```python
from build123d import *

# Parameters (mm, degrees)
SKETCH1_R                       = 2.6
SKETCH1_R_2                     = 1.5
SKETCH1_W                       = 44.817241247
SKETCH1_H                       = 25.097655098
BOSS_EXTRUDE1_DEPTH             = 5
SKETCH2_R                       = 5
SKETCH2_R_2                     = 2.6
BOSS_EXTRUDE2_DEPTH             = 12
BOSS_EXTRUDE2_DIRECTION_2_REACH = 102.099
BOSS_EXTRUDE3_START             = -10
SKETCH3_R                       = 2.6
BOSS_EXTRUDE3_DEPTH             = 10


with BuildPart() as part:
    # Sketch1 → Boss-Extrude1 (new body)
    with BuildSketch(Plane.XY):
        with BuildLine():
            ThreePointArc((-87.127451531, -22.124820062), (-86.163911981, -24.765644938), (-83.600914186, -25.920377287))
            ThreePointArc((-83.600914186, -25.920377287), (-47.661538714, -29.763777863), (-13.512307499, -17.921462012))
            ThreePointArc((-13.512307499, -17.921462012), (-10.952947302, -16.861340184), (-9.892825615, -14.301979929))
            ThreePointArc((-9.892825615, -14.301979929), (8.007659225, 5.698020071), (-9.892825615, 25.698020071))
            ThreePointArc((-9.892825615, 25.698020071), (-10.952947373, 28.257380397), (-13.512307698, 29.317502154))
            ThreePointArc((-13.512307698, 29.317502154), (-47.63265011, 41.014505592), (-83.512307597, 37.317502154))
            ThreePointArc((-83.512307597, 37.317502154), (-86.071667988, 36.257380433), (-87.131789782, 33.698020071))
            ThreePointArc((-87.131789782, 33.698020071), (-90.927012387, 5.786304892), (-87.127451531, -22.124820062))
        make_face()
        with Locations((-83.512307698, -22.301979929)):
            Circle(SKETCH1_R, mode=Mode.SUBTRACT)
        with Locations((-83.512307698, 33.698020071)):
            Circle(SKETCH1_R, mode=Mode.SUBTRACT)
        with Locations((-13.512307698, 25.698020071)):
            Circle(SKETCH1_R, mode=Mode.SUBTRACT)
        with Locations((-13.512307698, -14.301979929)):
            Circle(SKETCH1_R, mode=Mode.SUBTRACT)
        with Locations((-85.16722268, 22.0113147)):
            Circle(SKETCH1_R_2, mode=Mode.SUBTRACT)
        with Locations((-85.523935714, -6.702744554)):
            Circle(SKETCH1_R_2, mode=Mode.SUBTRACT)
        with Locations((-6.064210345, 17.314888474)):
            Circle(SKETCH1_R_2, mode=Mode.SUBTRACT)
        with Locations((-5.445296778, -4.691116539)):
            Circle(SKETCH1_R_2, mode=Mode.SUBTRACT)
        with BuildLine():
            Line((-79.892825615, -14.301980328), (-79.892825615, -22.301979929))
            ThreePointArc((-79.892825615, -22.301979929), (-47.851158005, -23.48878534), (-17.131789782, -14.301980328))
            Line((-17.131789782, -14.301980328), (-79.892825615, -14.301980328))
        make_face(mode=Mode.SUBTRACT)
        with BuildLine():
            Line((-79.892825615, 33.698019868), (-79.892825615, 25.698020071))
            Line((-79.892825615, 25.698020071), (-17.131789782, 25.698020071))
            ThreePointArc((-17.131789782, 25.698020071), (-47.634119077, 36.587523584), (-79.892825615, 33.698019868))
        make_face(mode=Mode.SUBTRACT)
        with Locations((-48.117941597, 5.846082995)):
            Rectangle(SKETCH1_W, SKETCH1_H, mode=Mode.SUBTRACT)
    extrude(amount=BOSS_EXTRUDE1_DEPTH)

    # Sketch2 → Boss-Extrude2 (add)
    # profile 1 of 4: a face of its own
    with BuildSketch(Plane(origin=(0, 0, 0), x_dir=(-1, 0, 0), z_dir=(0, 0, -1))):
        with Locations((13.512307698, 25.698020071)):
            Circle(SKETCH2_R)
        with Locations((13.512307698, 25.698020071)):
            Circle(SKETCH2_R_2, mode=Mode.SUBTRACT)
    # profile 2 of 4: a face of its own
    with BuildSketch(Plane(origin=(0, 0, 0), x_dir=(-1, 0, 0), z_dir=(0, 0, -1))):
        with Locations((83.512307698, 33.698020071)):
            Circle(SKETCH2_R)
        with Locations((83.512307698, 33.698020071)):
            Circle(SKETCH2_R_2, mode=Mode.SUBTRACT)
    # profile 3 of 4: a face of its own
    with BuildSketch(Plane(origin=(0, 0, 0), x_dir=(-1, 0, 0), z_dir=(0, 0, -1))):
        with Locations((83.512307698, -22.301979929)):
            Circle(SKETCH2_R)
        with Locations((83.512307698, -22.301979929)):
            Circle(SKETCH2_R_2, mode=Mode.SUBTRACT)
    # profile 4 of 4: a face of its own
    with BuildSketch(Plane(origin=(0, 0, 0), x_dir=(-1, 0, 0), z_dir=(0, 0, -1))):
        with Locations((13.512307698, -14.301979929)):
            Circle(SKETCH2_R)
        with Locations((13.512307698, -14.301979929)):
            Circle(SKETCH2_R_2, mode=Mode.SUBTRACT)
    extrude(amount=BOSS_EXTRUDE2_DEPTH)

    # Boss-Extrude2 direction 2: up to this face of the body (flat: up to its plane)
    boss_extrude2_direction_2_end = Plane(part.part.faces().sort_by_distance((-86.07433416, -24.682416176, 5))[0])
    # Sketch2 → Boss-Extrude2 direction 2 (add, up to the picked face)
    with BuildSketch(Plane(origin=(0, 0, 0), x_dir=(-1, 0, 0), z_dir=(0, 0, -1)), mode=Mode.PRIVATE) as boss_extrude2_direction_2_sk1:
        with Locations((13.512307698, 25.698020071)):
            Circle(SKETCH2_R)
        with Locations((13.512307698, 25.698020071)):
            Circle(SKETCH2_R_2, mode=Mode.SUBTRACT)
    boss_extrude2_direction_2_tool1 = split(extrude(boss_extrude2_direction_2_sk1.sketch, amount=-BOSS_EXTRUDE2_DIRECTION_2_REACH, mode=Mode.PRIVATE), bisect_by=boss_extrude2_direction_2_end, keep=Keep.BOTH, mode=Mode.PRIVATE)
    # Sketch2 → Boss-Extrude2 direction 2 (add, up to the picked face)
    with BuildSketch(Plane(origin=(0, 0, 0), x_dir=(-1, 0, 0), z_dir=(0, 0, -1)), mode=Mode.PRIVATE) as boss_extrude2_direction_2_sk2:
        with Locations((83.512307698, 33.698020071)):
            Circle(SKETCH2_R)
        with Locations((83.512307698, 33.698020071)):
            Circle(SKETCH2_R_2, mode=Mode.SUBTRACT)
    boss_extrude2_direction_2_tool2 = split(extrude(boss_extrude2_direction_2_sk2.sketch, amount=-BOSS_EXTRUDE2_DIRECTION_2_REACH, mode=Mode.PRIVATE), bisect_by=boss_extrude2_direction_2_end, keep=Keep.BOTH, mode=Mode.PRIVATE)
    # Sketch2 → Boss-Extrude2 direction 2 (add, up to the picked face)
    with BuildSketch(Plane(origin=(0, 0, 0), x_dir=(-1, 0, 0), z_dir=(0, 0, -1)), mode=Mode.PRIVATE) as boss_extrude2_direction_2_sk3:
        with Locations((83.512307698, -22.301979929)):
            Circle(SKETCH2_R)
        with Locations((83.512307698, -22.301979929)):
            Circle(SKETCH2_R_2, mode=Mode.SUBTRACT)
    boss_extrude2_direction_2_tool3 = split(extrude(boss_extrude2_direction_2_sk3.sketch, amount=-BOSS_EXTRUDE2_DIRECTION_2_REACH, mode=Mode.PRIVATE), bisect_by=boss_extrude2_direction_2_end, keep=Keep.BOTH, mode=Mode.PRIVATE)
    # Sketch2 → Boss-Extrude2 direction 2 (add, up to the picked face)
    with BuildSketch(Plane(origin=(0, 0, 0), x_dir=(-1, 0, 0), z_dir=(0, 0, -1)), mode=Mode.PRIVATE) as boss_extrude2_direction_2_sk4:
        with Locations((13.512307698, -14.301979929)):
            Circle(SKETCH2_R)
        with Locations((13.512307698, -14.301979929)):
            Circle(SKETCH2_R_2, mode=Mode.SUBTRACT)
    boss_extrude2_direction_2_tool4 = split(extrude(boss_extrude2_direction_2_sk4.sketch, amount=-BOSS_EXTRUDE2_DIRECTION_2_REACH, mode=Mode.PRIVATE), bisect_by=boss_extrude2_direction_2_end, keep=Keep.BOTH, mode=Mode.PRIVATE)
    add(boss_extrude2_direction_2_tool1.solids().sort_by(Axis((-8.653729, 25.69802, 0), (0, 0, 1)))[0])
    add(boss_extrude2_direction_2_tool2.solids().sort_by(Axis((-78.653729, 33.69802, 0), (0, 0, 1)))[0])
    add(boss_extrude2_direction_2_tool3.solids().sort_by(Axis((-78.653729, -22.30198, 0), (0, 0, 1)))[0])
    add(boss_extrude2_direction_2_tool4.solids().sort_by(Axis((-8.653729, -14.30198, 0), (0, 0, 1)))[0])

    # Sketch3 → Boss-Extrude3 (add)
    with BuildSketch(Plane.XY.offset(5).offset(BOSS_EXTRUDE3_START)):
        with Locations(Location((-83.512307698, 33.698020071, 0), (0, 0, 180))):
            Circle(SKETCH3_R)
        with Locations(Location((-13.512307698, 25.698020071, 0), (0, 0, 180))):
            Circle(SKETCH3_R)
        with Locations(Location((-13.512307698, -14.301979929, 0), (0, 0, 180))):
            Circle(SKETCH3_R)
        with Locations(Location((-83.512307698, -22.301979929, 0), (0, 0, 180))):
            Circle(SKETCH3_R)
    extrude(amount=BOSS_EXTRUDE3_DEPTH)


solid = part.part
```
Geometry: final body of the model. Coordinates: model frame, mm. A direction names the side the tool comes from. Coordinates: 2 decimals unless noted, no trailing zeros. Order: outer loops, then holes, each group sorted by start corner. A loop starts at its lowest first (then second) coordinate and runs counter-clockwise, first axis right, second up. Notation, with made-up numbers: (2.25, -39.5) - (26.25, -39.5) arc R11 ccw to (26.25, -24.5) - close; hole circle Ø9 at (26, 54). An arc over 180 degrees is marked (long way). Return JSON: item names as keys, results as strings. Group by question number.
1. Cut plane A-A (x = -66.5). Output: boundary loops of the cut face in (y, z), plus the area to 3 significant figures.
2. Pull-direction query (X, two-part tool) for faces 1 (the face through (-83, -22, -5)), 2 (the face through (-86, 32, -12)), 3 (the face through (-13, 26, -5)), 4 (the face through (8.004, 5.306, 2.465)); classes: pulls with the +X half, pulls with the -X half, needs draft (parallel to the pull), parting line crosses it, or undercut.
3. Set-up query: faces 5 (the face through (-15.99, 26.48, -8.45)), 6 (the face through (-16, -16, -12)), 7 (the face through (-79.893, 28, 2)). Return all of +Z, -Z, +X, -X, +Y, -Y with unobstructed straight access to the full face (end or side cutting, diameter ignored); none if empty.
4. Cut plane D-D (x = -54.5). Output: boundary loops of the cut face in (y, z), plus the area to 3 significant figures.
5. Material intervals for line 1 along Y through (x, z) = (-49, 1); line 2 along Y through (x, z) = (-78, 1.5); line 3 along Y through (x, z) = (-84, -5.5), sorted ascending. Write a range as [from, to].
6. Cut plane B-B (z = -8). Output: boundary loops of the cut face in (x, y), plus the area to 3 significant figures.
7. Cut plane C-C (y = 14). Output: boundary loops of the cut face in (x, z).
8. Pin query (flat end, axial travel): pin 1 (4 mm diameter, centred on x = -51, z = 3, fed in from -Y); pin 2 (10 mm diameter, centred on x = -31, z = 0.5, fed in from -Y); pin 3 (1 mm diameter, centred on y = 24, z = -3.5, fed in from -X); pin 4 (8 mm diameter, centred on y = -2.5, z = -4.5, fed in from +X). Return the tip coordinate at first contact, or that it passes through.
Resolved:
{
 "1": {"outline": "(-29.76, 0) - (-24.08, 0) - (-24.08, 5) - (-29.76, 5) - close; (-14.3, 0) - (-6.7, 0) - (-6.7, 5) - (-14.3, 5) - close; (18.39, 0) - (25.7, 0) - (25.7, 5) - (18.39, 5) - close; (36.62, 0) - (41.04, 0) - (41.04, 5) - (36.62, 5) - close", "area": "125 mm²"},
 "2": {"face 1": "undercut", "face 2": "needs draft", "face 3": "undercut", "face 4": "pulls with the +X half"},
 "3": {"face 5": "-Z", "face 6": "-Z, +X, -X, +Y, -Y", "face 7": "+Z, -Z"},
 "4": {"outline": "(-30.26, 0) - (-24.11, 0) - (-24.11, 5) - (-30.26, 5) - close; (-14.3, 0) - (-6.7, 0) - (-6.7, 5) - (-14.3, 5) - close; (18.39, 0) - (25.7, 0) - (25.7, 5) - (18.39, 5) - close; (37.15, 0) - (41.52, 0) - (41.52, 5) - (37.15, 5) - close", "area": "127 mm²"},
 "5": {"line 1": "y = [-29.91, -23.63], [-14.3, -6.7], [18.39, 25.7], [36.75, 41.16]", "line 2": "y = [-27.6, -22.67], [-14.3, 25.7], [34.27, 38.93]", "line 3": "y = [-27.28, -24.86], [-19.75, -17.33], [28.72, 31.14], [36.25, 38.67]"},
 "6": {"outline": "circle Ø10 at (-83.51, -22.3); circle Ø10 at (-83.51, 33.7); circle Ø10 at (-13.51, -14.3); circle Ø10 at (-13.51, 25.7); hole circle Ø5.2 at (-83.51, -22.3); hole circle Ø5.2 at (-83.51, 33.7); hole circle Ø5.2 at (-13.51, -14.3); hole circle Ø5.2 at (-13.51, 25.7)", "area": "229 mm²"},
 "7": {"outline": "(-90.6, 0) - (-70.53, 0) - (-70.53, 5) - (-90.6, 5) - close; (-25.71, 0) - (6.22, 0) - (6.22, 5) - (-25.71, 5) - close"},
 "8": {"pin 1": "stops at y = -30.2", "pin 2": "stops at y = -27.58", "pin 3": "stops at x = -18.37", "pin 4": "passes through"}
}
